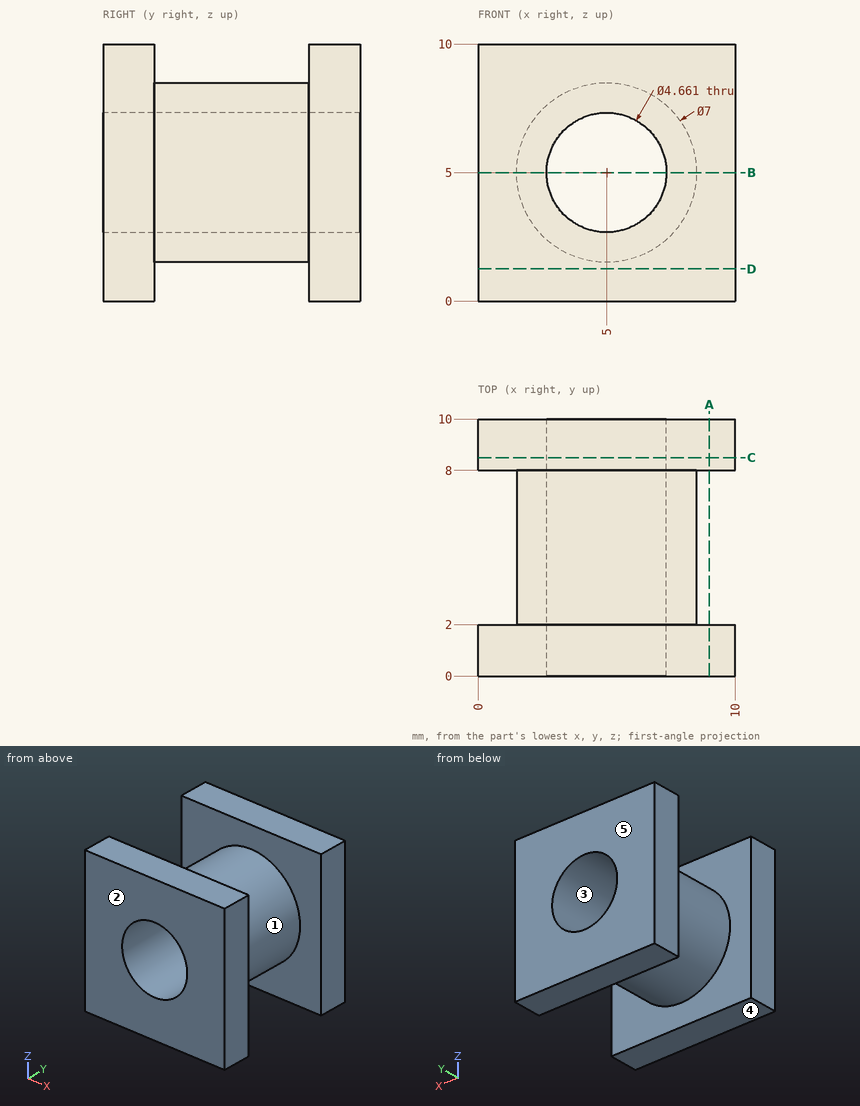
The drawing under review shows one solid part. Ordinate dimensions are in mm from its lowest x, y, z. A direction names the side the tool comes from. Round coordinates to 2 decimals unless told otherwise and drop trailing zeros. Write each loop counter-clockwise with the first axis right and the second up, starting at its lowest first coordinate (ties: lowest second). Pieces come first, ordered by that corner, then holes. Notation, with made-up numbers: (-28.75, 82.5) - (-18.75, 82.5) arc R36 ccw to (-18.75, 119.5) - close; hole circle Ø9 at (52, 59.5). An arc over 180 degrees is marked (long way). Put each result on its own line as item: value.
Q1. We need section C-C (y = 8.5). Give the boundary of the cut face in (x, z), and give its area (3 significant figures).
Solved:
outline: (0, 0) - (10, 0) - (10, 10) - (0, 10) - close; hole circle Ø4.66 at (5, 5)
area: 82.9 mm2
Q2. Machinability: for the marked faces 1 and 2, which of the approach directions +Z, -Z, +X, -X, +Y, -Y give a long, thin tool a straight path to every point of the face, cutting with its end or side? Answer none if there is none.
Solved:
face 1: none
face 2: +Z, -Z, +X, -X, -Y
Q3. Wall thickness on probe 1 along X at (y, z) = (3.75, 5); probe 2 along Y at (x, z) = (9.25, 6.25); probe 3 along Z at (x, y) = (4.5, 9.25): over which ranges is each line inside the solid? List them lowest first.
Solved:
probe 1: x = 1.5 to 2.67, 7.33 to 8.5
probe 2: y = 0 to 2, 8 to 10
probe 3: z = 0 to 2.72, 7.28 to 10
Q4. Insertion check: pin 1 Ø3.5 at (x, z) = (5, 5) entering from +Y. The pin has a flat end and moves straight along its axis. Give the tip position at first contact, or say it passes through.
Solved:
pin 1: passes through
Q5. We need section B-B (z = 5). Give the boundary of the cut face in (x, y).
Solved:
outline: (0, 0) - (2.67, 0) - (2.67, 10) - (0, 10) - (0, 8) - (1.5, 8) - (1.5, 2) - (0, 2) - close; (7.33, 0) - (10, 0) - (10, 2) - (8.5, 2) - (8.5, 8) - (10, 8) - (10, 10) - (7.33, 10) - close
Q6. We need section A-A (x = 9). Give the boundary of the cut face in (y, z), and give its area (3 significant figures).
Solved:
outline: (0, 0) - (2, 0) - (2, 10) - (0, 10) - close; (8, 0) - (10, 0) - (10, 10) - (8, 10) - close
area: 40.0 mm2
Q7. We need section D-D (z = 1.25). Give the boundary of the cut face in (x, y), and give its area (3 significant figures).
Solved:
outline: (0, 0) - (10, 0) - (10, 2) - (0, 2) - close; (0, 8) - (10, 8) - (10, 10) - (0, 10) - close
area: 40.0 mm2
Q8. Mouldability with a two-part tool opening along Z and no side actions: class the marked faces 3, 4 and 5 as released by +Z, released by -Z, zero draft, split by the parting line, or undercut.
Solved:
face 3: undercut
face 4: released by -Z
face 5: zero draft
